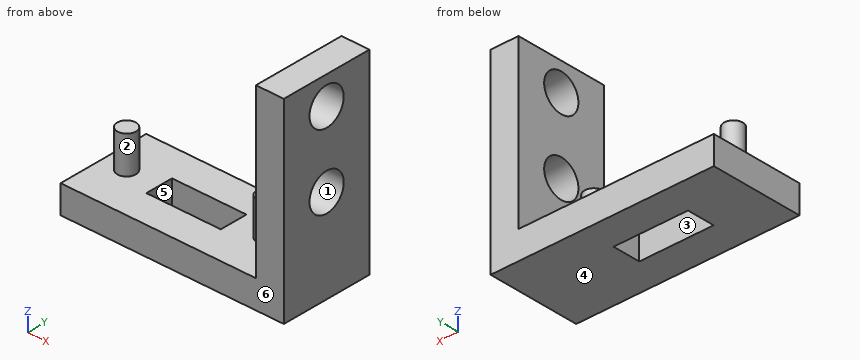
from build123d import *

# Parameters (mm, degrees)
F1_DEPTH = 10
F2_R     = 1
F3_DEPTH = 4
F4_W     = 8
F4_H     = 3
F5_DEPTH = 25
F6_R     = 2
F7_DEPTH = 25


with BuildPart() as f1:
    # F0 (on Front) → F1 (new body)
    with BuildSketch(Plane.XZ):
        Polygon((-24, 0), (0, 0), (0, 21), (-3, 21), (-3, 3), (-24, 3), align=None)
    extrude(amount=F1_DEPTH)

    # F2 (on face) → F3 (join)
    with BuildSketch(Plane.XY.offset(3)):
        with Locations((-21.5, -5)):
            Circle(F2_R)
        with Locations((-6.5, -5)):
            Circle(F2_R)
    extrude(amount=F3_DEPTH)

    # F4 (on face) → F5 (cut)
    with BuildSketch(Plane.XY.offset(3)):
        with Locations((-14, -5)):
            Rectangle(F4_W, F4_H)
    extrude(amount=-F5_DEPTH, mode=Mode.SUBTRACT)

    # F6 (on face) → F7 (cut)
    with BuildSketch(Plane(origin=(-3, 0, 0), x_dir=(0, -1, 0), z_dir=(-1, 0, 0))):
        with Locations((5, 18)):
            Circle(F6_R)
        with Locations((5, 10)):
            Circle(F6_R)
    extrude(amount=-F7_DEPTH, mode=Mode.SUBTRACT)


solid = f1.part
Geometry: final body of the model. Coordinates: model frame, mm. Face numbers are marked on the shaded views. A direction names the side the tool comes from. Coordinates: 2 decimals unless noted, no trailing zeros. Loops run counter-clockwise (first coordinate to the right, second up) from the corner with the lowest first, then second, coordinate; pieces in that order, holes last. Notation, with made-up numbers: (27.5, 67.5) - (57.5, 67.5) arc R20 cw to (57.5, 91.5) - close; hole circle Ø7 at (-38, 86.5). An arc over 180 degrees is marked (long way). Put each result on its own line as item: value. Start each with the question number.
Q1. Cut plane D-D, the plane x = -2.25. Return loops of the section in (y, z), and give its area (3 significant figures).
Q2. Cut plane A-A, the plane y = -5. Return loops of the section in (x, z).
Q3. Pull-direction query (Y, two-part tool) for the marked faces 4, 5 and 6; classes: released by +Y, released by -Y, zero draft, split by the parting line, or undercut.
Q4. Cut plane B-B, the plane z = 10. Return loops of the section in (x, y), and give its area (3 significant figures).
Q5. Line query: line 1 (Z direction, x = -0.8, y = -5); line 2 (X direction, y = -6, z = 1.5); line 3 (X direction, y = -3, z = 4.5). Output: solid intervals per line, ascending.
Q6. Pin query (flat end, axial travel): pin 1 Ø1.6 at (x, y) = (-7, -4.5) entering from +Z; pin 2 Ø5 at (y, z) = (-6.5, 8) entering from -X; pin 3 Ø5 at (x, y) = (-11.5, -4.5) entering from +Z. Return the tip coordinate at first contact, or that it passes through.
Q7. Cut plane C-C, the plane x = -6.5. Return loops of the section in (y, z).
Q8. Set-up query: the marked faces 1, 2 and 3. Return all of +Z, -Z, +X, -X, +Y, -Y with unobstructed straight access to the full face (end or side cutting, diameter ignored); none if empty.
Filled sheet:
1. outline: (-10, 0) - (0, 0) - (0, 21) - (-10, 21) - close; hole circle Ø4 at (-5, 10); hole circle Ø4 at (-5, 18)
1. area: 185 mm²
2. outline: (-24, 0) - (-18, 0) - (-18, 3) - (-20.5, 3) - (-20.5, 7) - (-22.5, 7) - (-22.5, 3) - (-24, 3) - close; (-10, 0) - (0, 0) - (0, 8) - (-3, 8) - (-3, 3) - (-5.5, 3) - (-5.5, 7) - (-7.5, 7) - (-7.5, 3) - (-10, 3) - close; (-3, 12) - (0, 12) - (0, 16) - (-3, 16) - close; (-3, 20) - (0, 20) - (0, 21) - (-3, 21) - close
3. face 4: zero draft
3. face 5: undercut
3. face 6: released by -Y
4. outline: (-3, -10) - (0, -10) - (0, -7) - (-3, -7) - close; (-3, -3) - (0, -3) - (0, 0) - (-3, 0) - close
4. area: 18.0 mm²
5. line 1: 0 to 8, 12 to 16, 20 to 21
5. line 2: -24 to -18, -10 to 0
5. line 3: -3 to 0
6. pin 1: z = 7
6. pin 2: x = -22.5
6. pin 3: z = 3
7. outline: (-10, 0) - (0, 0) - (0, 3) - (-4, 3) - (-4, 7) - (-6, 7) - (-6, 3) - (-10, 3) - close
8. face 1: +X, -X
8. face 2: +Z
8. face 3: +Z, -Z
